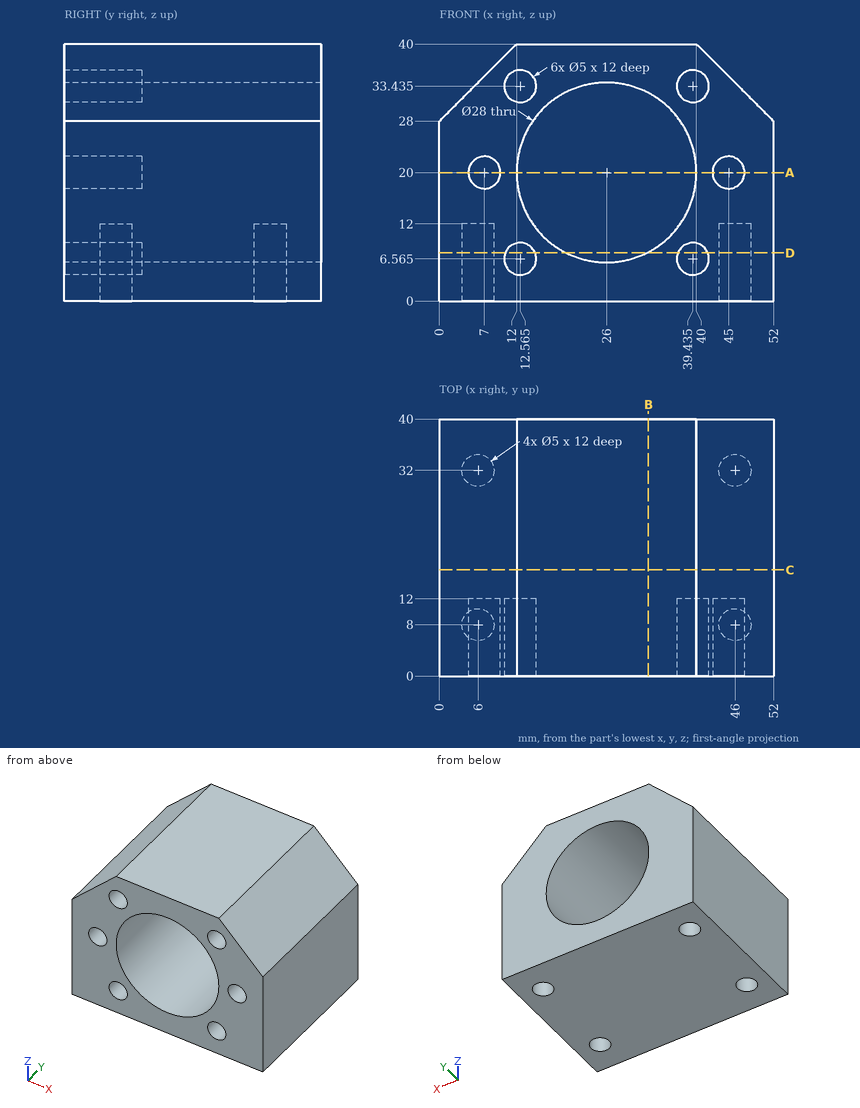
Source: three-view drawing plus pictorial views. Frame: mm from the lowest corner of the part. Round coordinates to 2 decimals unless told otherwise and drop trailing zeros. Order: outer loops, then holes, each group sorted by start corner. A loop starts at its lowest first (then second) coordinate and runs counter-clockwise, first axis right, second up. Notation, with made-up numbers: (-9.5, 21) -> (25.5, 21) arc R28 ccw to (25.5, 58) -> close; hole circle Ø4 at (72, 3). An arc over 180 degrees is marked (long way). Use one line per item in the form item = value. Start each with the question number.
1. Line query: probe 1 along Y at (x, z) = (6, 3.75); probe 2 along X at (y, z) = (8, 7); probe 3 along Z at (x, y) = (26, 27). Output: solid intervals per line, ascending.
2. Cut plane D-D (z = 7.5). Return the cut outline in (x, y).
3. Cut plane A-A (z = 20). Return the cut outline in (x, y), then the cut area to 3 significant figures.
4. Cut plane C-C (y = 16.5). Return the cut outline in (x, z).
5. Pin query (flat end, axial travel): pin 1 Ø1.5 at (x, z) = (7, 19.5) entering from -Y; pin 2 Ø6.5 at (x, y) = (46, 8) entering from +Z; pin 3 Ø8 at (x, y) = (6, 8) entering from +Z. Return the tip coordinate at first contact, or that it passes through.
6. Cut plane B-B (x = 32.5). Return the cut outline in (y, z).
Solution:
q1.probe_1 = 0 to 5.5, 10.5 to 29.5, 34.5 to 40
q1.probe_2 = 0 to 3.5, 8.5 to 10.1, 15.03 to 20.8, 31.2 to 36.97, 41.9 to 43.5, 48.5 to 52
q1.probe_3 = 0 to 6, 34 to 40
q2.outline = (0, 0) -> (10.25, 0) -> (10.25, 12) -> (14.88, 12) -> (14.88, 0) -> (19.7, 0) -> (19.7, 40) -> (0, 40) -> close; (32.3, 0) -> (37.12, 0) -> (37.12, 12) -> (41.75, 12) -> (41.75, 0) -> (52, 0) -> (52, 40) -> (32.3, 40) -> close; hole circle Ø5 at (6, 8); hole circle Ø5 at (6, 32); hole circle Ø5 at (46, 8); hole circle Ø5 at (46, 32)
q3.outline = (0, 0) -> (4.5, 0) -> (4.5, 12) -> (9.5, 12) -> (9.5, 0) -> (12, 0) -> (12, 40) -> (0, 40) -> close; (40, 0) -> (42.5, 0) -> (42.5, 12) -> (47.5, 12) -> (47.5, 0) -> (52, 0) -> (52, 40) -> (40, 40) -> close
q3.area = 840 mm^2
q4.outline = (0, 0) -> (52, 0) -> (52, 28) -> (40, 40) -> (12, 40) -> (0, 28) -> close; hole circle Ø28 at (26, 20)
q5.pin_1 = 12
q5.pin_2 = 37.25
q5.pin_3 = 38
q6.outline = (0, 0) -> (40, 0) -> (40, 7.6) -> (0, 7.6) -> close; (0, 32.4) -> (40, 32.4) -> (40, 40) -> (0, 40) -> close
